Autodesk Inventor part; units mm, degrees
ref_plane "YZ Plane" through (0, 0, 0) normal (1, 0, 0) x (0, 1, 0)
ref_plane "XZ Plane" through (0, 0, 0) normal (0, 1, 0) x (-1, 0, 0)
ref_plane "XY Plane" through (0, 0, 0) normal (0, 0, 1) x (1, 0, 0)
sketch "Szkic1" plane through (0, 0, 0) normal (0, 0, 1) x (1, 0, 0)
  line L0 (-28.5, -96.5) -> (28.5, -96.5)
  line L1 (28.5, -96.5) -> (28.5, 33.5)
  line L2 (28.5, 33.5) -> (-28.5, 33.5)
  line L3 (-28.5, 33.5) -> (-28.5, -96.5)
  line L4 (-28.5, -96.5) -> (28.5, 33.5) construction
  line L5 (28.5, -96.5) -> (-28.5, 33.5) construction
  line L6 (0, -96.5) -> (0, 33.5) construction
  line L7 (-26.5, 33.5) -> (26.5, 33.5)
  line L8 (26.5, -23.5) -> (-26.5, -23.5)
  line L9 (0, -23.5) -> (0, 33.5) construction
  point P0 (0, -31.5)
  dimension "d0" = 57
  dimension "d1" = 130
extrude "Wyciągnięcie proste1" add sketch "Szkic1" along normal blind 2
sketch "Szkic2" plane through (0, 0, 0) normal (0, 0, -1) x (-1, 0, 0)
  circle A0 centre (0, 5) radius 5
  circle A1 centre (0, 5) radius 19.05
  point P0 (0, 0)
extrude "Wyciągnięcie proste2" cut sketch "Szkic2" against normal blind 10 contours A0 | A1
sketch "Szkic3" plane through (0, 0, 0) normal (0, 0, -1) x (-1, 0, 0)
  circle A0 centre (-23.57, -18.57) radius 2.5
  circle A1 centre (23.57, -18.57) radius 2.5
  circle A2 centre (23.57, 28.57) radius 2.5
  circle A3 centre (-23.57, 28.57) radius 2.5
  point P0 (0, 0)
extrude "Wyciągnięcie proste3" cut sketch "Szkic3" against normal blind 10
ref_plane "Płaszczyzna konstrukcyjna1" through (18.5, -96.5, 0) normal (1, 0, 0) x (0, 0, -1)
sketch "Szkic5" plane through (18.5, -96.5, 0) normal (1, 0, 0) x (0, 0, -1)
  line L0 (-2, 0) -> (-27, 0)
  line L1 (-27, 0) -> (-2, 25)
  line L2 (-2, 0) -> (-2, 25)
  point P0 (0, 66.5)
  dimension "d14" = 25
extrude "Wyciągnięcie proste5" add sketch "Szkic5" against normal blind 2
mirror "Odbicie lustrzane1" about plane through (0, 0, 0) normal (1, 0, 0) of "Wyciągnięcie proste5"
properties part number "stepper_console_large"
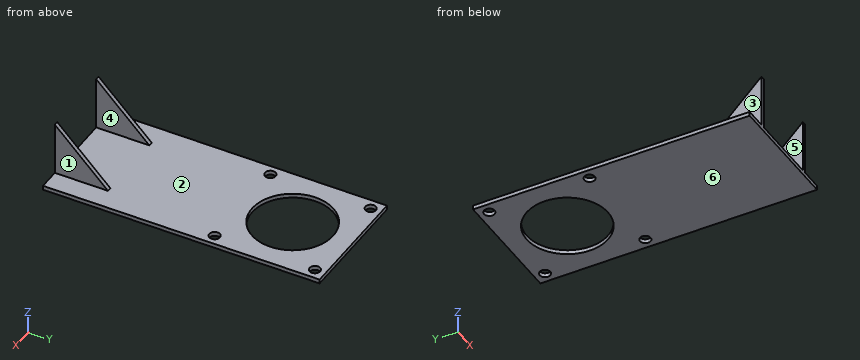
Verification items for the finished model (mm, model axes). Face numbers are marked on the shaded views. A direction names the side the tool comes from. Give positions to 0.01 mm unless a question says otherwise; leave off trailing zeros. Order: outer loops, then holes, each group sorted by start corner. A loop starts at its lowest first (then second) coordinate and runs counter-clockwise, first axis right, second up. Notation, with made-up numbers: M 37.5,-28 L 45.5,-28 A16 ccw 45.5,-23 Z; hole C 31.25,43 d3. An arc over 180 degrees is marked long. Return JSON: item names as keys, results as strings. Group by question number.
1) Mould release check, pull along X, two halves, no side actions. Record for the marked faces 1, 2, 3 and 4: pulls with the +X half, pulls with the -X half, needs draft (parallel to the pull), parting line crosses it, or undercut.
2) Go/stop test with flat-tipped pins: pin 1 Ø5 at (x, z) = (-15.5, 11.5) entering from +Y; pin 2 Ø3 at (x, y) = (11.5, -29.5) entering from +Z; pin 3 Ø4 at (x, y) = (-23.57, -18.57) entering from +Z. Record where each tip stops, or that it passes through.
3) Section check A-A on y = -18.57. Record the cut outline in (x, z).
4) Section check B-B on z = 17.75. Record the cut outline in (x, y), and give its area (3 significant figures).
5) Section check C-C on x = 0. Record the cut outline in (y, z), and give its area (3 significant figures).
6) Scan lines: line 1 (Y direction, x = -23.57, z = 0.6); line 2 (X direction, y = -84.5, z = 6.25); line 3 (Y direction, x = 0, z = 1.15). Record each from-to range of solid material in increasing order.
7) Access from +Z, -Z, +X, -X, +Y, -Y to the whole of each face (thin tool, end or side, straight path). Record for the marked faces 5 and 6.
8) Section check D-D on x = 23.57. Record the cut outline in (y, z).
Answer block:
{
 "1": {"face 1": "pulls with the +X half", "face 2": "undercut", "face 3": "pulls with the -X half", "face 4": "undercut"},
 "2": {"pin 1": "stops at y = -78.71", "pin 2": "stops at z = 2", "pin 3": "passes through"},
 "3": {"outline": "M -28.5,0 L -26.07,0 L -26.07,2 L -28.5,2 Z; M -21.07,0 L 21.07,0 L 21.07,2 L -21.07,2 Z; M 26.07,0 L 28.5,0 L 28.5,2 L 26.07,2 Z"},
 "4": {"outline": "M -18.5,-96.5 L -16.5,-96.5 L -16.5,-87.25 L -18.5,-87.25 Z; M 16.5,-96.5 L 18.5,-96.5 L 18.5,-87.25 L 16.5,-87.25 Z", "area": "37.0 mm^2"},
 "5": {"outline": "M -96.5,0 L -14.05,0 L -14.05,2 L -96.5,2 Z; M 24.05,0 L 33.5,0 L 33.5,2 L 24.05,2 Z", "area": "184 mm^2"},
 "6": {"line 1": "y = -96.5 to -21.07, -16.07 to 26.07, 31.07 to 33.5", "line 2": "x = -18.5 to -16.5, 16.5 to 18.5", "line 3": "y = -96.5 to -14.05, 24.05 to 33.5"},
 "7": {"face 5": "+Z, +Y, -Y", "face 6": "-Z, +X, -X, +Y, -Y"},
 "8": {"outline": "M -96.5,0 L -21.07,0 L -21.07,2 L -96.5,2 Z; M -16.07,0 L 26.07,0 L 26.07,2 L -16.07,2 Z; M 31.07,0 L 33.5,0 L 33.5,2 L 31.07,2 Z"}
}
